Read the model definition and answer for the solid it produces. Units are mm, in the model's axes. A direction names the side the tool comes from. Coordinates: 2 decimals unless noted, no trailing zeros. Loops run counter-clockwise (first coordinate to the right, second up) from the corner with the lowest first, then second, coordinate; pieces in that order, holes last. Notation, with made-up numbers: (13, 38) -> (68, 38) arc R24 cw to (68, 72) -> close; hole circle Ø2 at (65, 15.25). An arc over 180 degrees is marked (long way). Answer as a JSON object with one key per item and string values. Group by question number.
Q1. Each of these flat-tipped pins is pushed along its axis until it touches: P1, Ø6, axis at x = 20.5, y = -10, coming from the +Z side; P2, Ø2, axis at y = -22.5, z = -13.5, coming from the -X side; P3, Ø8.5, axis at x = -4.07, y = -19.05, coming from the -Z side; P4, Ø1, axis at x = -5.5, z = -4.5, coming from the +Y side. Where does it stop, or does it pass through?
Q2. Straight lines are drawn through the part: line 1 along X through (y, z) = (-6.35, -2.75); line 2 along X through (y, z) = (-19.05, -2.5); line 3 along X through (y, z) = (-19.05, -3.5). For each, find the intervals that lie inside material, in ascending order. Write a range as [from, to].
Q3. For faces 5 (the cylindrical face through (-1.04, -5.4, -3.09)), 6 (the cylindrical face through (30.29, -12.52, -0.31)), 7 (the flat face through (38, -13, -3.175)), determine the directions among +Z, -Z, +X, -X, +Y, -Y from which every point of the face is accessible in a straight line to the end or side of a thin tool.
Q4. Determine the mould class of faces 1 (the cylindrical face through (-0.31, -12.52, -0.33)), 2 (the cylindrical face through (30.86, -18.91, -3.09)), 3 (the cylindrical face through (32.956, -12.65, -3.427)), 4 (the flat face through (-7, -13, 0)) for opening direction X: released by +X, released by -X, zero draft, split by the parting line, or undercut.
Q5. The part is cut by section B-B on z = -6.5. Write down the section's boundary in (x, y) (3 decimals).
Q6. The part is cut by section C-C on x = -4.5. Write down the section's boundary in (y, z) (3 decimals), and give its area (3 significant figures).
Q7. The part is cut by section A-A on y = -19.05. Write down the section's boundary in (x, z) (3 decimals), and give its area (3 significant figures).
from build123d import *

# Parameters (mm, degrees)
BOSS_EXTRUDE1_DEPTH = 25.4
SKETCH3_R           = 3.175
CUT_EXTRUDE1_DEPTH  = 51.78354129
FILLET1_R           = 1.27


with BuildPart() as part:
    # Sketch2 → Boss-Extrude1 (new body)
    with BuildSketch(Plane(origin=(0, 0, 0), x_dir=(1, 0, 0), z_dir=(0, 1, 0))):
        with BuildLine():
            Line((0, 0), (-10.419367303, 0))
            Line((-10.419367303, 0), (-10.419367303, 3.175))
            Line((-10.419367303, 3.175), (-2.762835284, 3.175))
            ThreePointArc((-2.762835284, 3.175), (14.980632697, 17.413), (32.724100678, 3.175))
            Line((32.724100678, 3.175), (40.380632697, 3.175))
            Line((40.380632697, 3.175), (40.380632697, 0))
            Line((40.380632697, 0), (29.961265394, 0))
            ThreePointArc((29.961265394, 0), (14.980632697, 14.238), (0, 0))
        make_face()
    extrude(amount=-BOSS_EXTRUDE1_DEPTH)

    # Sketch3 → Cut-Extrude1 (cut, through all)
    with BuildSketch(Plane.XY):
        with Locations((-4.069367303, -6.35)):
            Circle(SKETCH3_R)
        with Locations((34.030632697, -6.35)):
            Circle(SKETCH3_R)
        with Locations((-4.069367303, -19.05)):
            Circle(SKETCH3_R)
        with Locations((34.030632697, -19.05)):
            Circle(SKETCH3_R)
    extrude(amount=-CUT_EXTRUDE1_DEPTH, mode=Mode.SUBTRACT)

    # Fillet1
    # the kernel refuses this fillet: 1.27 mm, written as the material it adds along each edge
    with BuildSketch(Plane(origin=(32.724100678, 0, -3.175), x_dir=(1, 0, 0), z_dir=(0, -1, 0))) as fillet1_piece_1_section:
        with BuildLine():
            CenterArc((0.991397271, -1.27), FILLET1_R, 90, 74.467738735)
            ThreePointArc((-0.232222111, -0.929918231), (-0.109979978, -0.466490187), (0, 0))
            Line((0, 0), (0.991397271, 0))
        make_face()
    fillet1_piece_1 = extrude(amount=5.934776002, mode=Mode.PRIVATE)
    fillet1_piece_1 = fillet1_piece_1 - Plane(origin=(34.030632697, -6.35, -3.384746049), x_dir=(1, 0, 0), z_dir=(0, 0, 1)) * Cylinder(3.175, 16, mode=Mode.PRIVATE)
    add(fillet1_piece_1)
    with BuildSketch(Plane(origin=(32.724100678, -19.465223998, -3.175), x_dir=(1, 0, 0), z_dir=(0, -1, 0))) as fillet1_piece_2_section:
        with BuildLine():
            CenterArc((0.991397271, -1.27), FILLET1_R, 90, 74.467738735)
            ThreePointArc((-0.232222111, -0.929918231), (-0.109979978, -0.466490187), (0, 0))
            Line((0, 0), (0.991397271, 0))
        make_face()
    fillet1_piece_2 = extrude(amount=5.934776002, mode=Mode.PRIVATE)
    fillet1_piece_2 = fillet1_piece_2 - Plane(origin=(34.030632697, -19.05, -3.384746046), x_dir=(1, 0, 0), z_dir=(0, 0, 1)) * Cylinder(3.175, 16, mode=Mode.PRIVATE)
    add(fillet1_piece_2)
    with BuildSketch(Plane(origin=(32.724100678, -6.765223998, -3.175), x_dir=(1, 0, 0), z_dir=(0, -1, 0))) as fillet1_piece_3_section:
        with BuildLine():
            CenterArc((0.991397271, -1.27), FILLET1_R, 90, 74.467738735)
            ThreePointArc((-0.232222111, -0.929918231), (-0.109979978, -0.466490187), (0, 0))
            Line((0, 0), (0.991397271, 0))
        make_face()
    fillet1_piece_3 = extrude(amount=11.869552004, mode=Mode.PRIVATE)
    fillet1_piece_3 = fillet1_piece_3 - Plane(origin=(34.030632697, -19.05, -3.384746051), x_dir=(1, 0, 0), z_dir=(0, 0, 1)) * Cylinder(3.175, 28, mode=Mode.PRIVATE)
    fillet1_piece_3 = fillet1_piece_3 - Plane(origin=(34.030632697, -6.35, -3.384746051), x_dir=(1, 0, 0), z_dir=(0, 0, 1)) * Cylinder(3.175, 28, mode=Mode.PRIVATE)
    add(fillet1_piece_3)
    with BuildSketch(Plane(origin=(-2.762835284, 0, -3.175), x_dir=(0.24228281636804117, 0, -0.9702056673163532), z_dir=(0, -1, 0))) as fillet1_piece_4_section:
        with BuildLine():
            CenterArc((0.991962675, -1.269558427), FILLET1_R, 91.510947972, 74.467738735)
            Line((-0.240198523, -0.96185925), (0, 0))
            ThreePointArc((0, 0), (0.479237682, -0.006319359), (0.958475365, 0))
        make_face()
    fillet1_piece_4 = extrude(amount=5.934776002, mode=Mode.PRIVATE)
    fillet1_piece_4 = fillet1_piece_4 - Plane(origin=(-4.069367303, -6.35, -3.384746045), x_dir=(1, 0, 0), z_dir=(0, 0, 1)) * Cylinder(3.175, 16, mode=Mode.PRIVATE)
    add(fillet1_piece_4)
    with BuildSketch(Plane(origin=(-2.762835284, -19.465223998, -3.175), x_dir=(0.24228281636804025, 0, -0.9702056673163533), z_dir=(0, -1, 0))) as fillet1_piece_5_section:
        with BuildLine():
            CenterArc((0.991962675, -1.269558427), FILLET1_R, 91.510947972, 74.467738735)
            Line((-0.240198523, -0.96185925), (0, 0))
            ThreePointArc((0, 0), (0.479237682, -0.006319359), (0.958475365, 0))
        make_face()
    fillet1_piece_5 = extrude(amount=5.934776002, mode=Mode.PRIVATE)
    fillet1_piece_5 = fillet1_piece_5 - Plane(origin=(-4.069367303, -19.05, -3.384746049), x_dir=(1, 0, 0), z_dir=(0, 0, 1)) * Cylinder(3.175, 16, mode=Mode.PRIVATE)
    add(fillet1_piece_5)
    with BuildSketch(Plane(origin=(-2.762835284, -6.765223998, -3.175), x_dir=(0.24228281636804025, 0, -0.9702056673163533), z_dir=(0, -1, 0))) as fillet1_piece_6_section:
        with BuildLine():
            CenterArc((0.991962675, -1.269558427), FILLET1_R, 91.510947972, 74.467738735)
            Line((-0.240198523, -0.96185925), (0, 0))
            ThreePointArc((0, 0), (0.479237682, -0.006319359), (0.958475365, 0))
        make_face()
    fillet1_piece_6 = extrude(amount=11.869552004, mode=Mode.PRIVATE)
    fillet1_piece_6 = fillet1_piece_6 - Plane(origin=(-4.069367303, -19.05, -3.38474605), x_dir=(1, 0, 0), z_dir=(0, 0, 1)) * Cylinder(3.175, 28, mode=Mode.PRIVATE)
    fillet1_piece_6 = fillet1_piece_6 - Plane(origin=(-4.069367303, -6.35, -3.38474605), x_dir=(1, 0, 0), z_dir=(0, 0, 1)) * Cylinder(3.175, 28, mode=Mode.PRIVATE)
    add(fillet1_piece_6)
    # the kernel refuses this fillet: 1.27 mm, written as the material it takes off along each edge
    with BuildSketch(Plane(origin=(29.961265394, 2.904944682, 0), x_dir=(1, 0, 0), z_dir=(0, -1, 0))) as fillet1_2_piece_1:
        with BuildLine():
            CenterArc((1.161977873, -1.27), FILLET1_R, 90, 82.825455624)
            ThreePointArc((-0.098078392, -1.111386601), (-0.038702449, -0.556605505), (0, 0))
            Line((0, 0), (1.161977873, 0))
        make_face()
    extrude(amount=31.209889363, mode=Mode.SUBTRACT)
    with BuildSketch(Plane(origin=(0, 2.904944682, 0), x_dir=(0.08790703364755922, 0, -0.996128683170647), z_dir=(0, -1, 0))) as fillet1_2_piece_2:
        with BuildLine():
            CenterArc((1.1629374, -1.269121421), FILLET1_R, 92.131332721, 82.825455624)
            Line((-0.102146028, -1.157479488), (0, 0))
            ThreePointArc((0, 0), (0.557852926, -0.010376919), (1.115705852, 0))
        make_face()
    extrude(amount=31.209889363, mode=Mode.SUBTRACT)


solid = part.part
Final values:
{
 "1": {"P1": "stops at z = -11.58", "P2": "stops at x = 2.55", "P3": "stops at z = -9.79", "P4": "passes through"},
 "2": {"line 1": "x = [-10.42, -7.24], [-0.89, 0.4], [29.56, 30.86], [37.21, 40.38]", "line 2": "x = [-10.42, -7.24], [-0.89, 0.34], [29.62, 30.86], [37.21, 40.38]", "line 3": "x = [-0.89, 0.6], [29.36, 30.86]"},
 "3": {"face 5": "+Z, -Z", "face 6": "+Z, +Y, -Y", "face 7": "-Z, +X, +Y, -Y"},
 "4": {"face 1": "undercut", "face 2": "undercut", "face 3": "released by +X", "face 4": "zero draft"},
 "5": {"outline": "(-1.681, -25.4) -> (1.856, -25.4) -> (1.856, 0) -> (-1.681, 0) -> (-1.681, -4.259) arc R3.175 cw to (-1.681, -8.441) -> (-1.681, -16.959) arc R3.175 cw to (-1.681, -21.141) -> close; (28.106, -25.4) -> (31.642, -25.4) -> (31.642, -21.141) arc R3.175 cw to (31.642, -16.959) -> (31.642, -8.441) arc R3.175 cw to (31.642, -4.259) -> (31.642, 0) -> (28.106, 0) -> close"},
 "6": {"outline": "(-25.4, -3.175) -> (-22.196, -3.175) -> (-22.196, 0) -> (-25.4, 0) -> close; (-15.904, -3.175) -> (-9.496, -3.175) -> (-9.496, 0) -> (-15.904, 0) -> close; (-3.204, -3.175) -> (0, -3.175) -> (0, 0) -> (-3.204, 0) -> close", "area": "40.7 mm2"},
 "7": {"outline": "(-10.419, -3.175) -> (-7.244, -3.175) -> (-7.244, 0) -> (-10.419, 0) -> close; (-0.894, -8.088) arc R18.175 ccw to (30.856, -8.088) -> (30.856, -0.029) arc R1.27 ccw to (29.863, -1.111) arc R15 cw to (0.098, -1.111) arc R1.27 ccw to (-0.894, -0.029) -> close; (37.206, -3.175) -> (40.381, -3.175) -> (40.381, 0) -> (37.206, 0) -> close", "area": "156 mm2"}
}
